For this review, take the finished solid that the model builds, in its own axes (mm). A direction names the side the tool comes from. Coordinates: 2 decimals unless noted, no trailing zeros. Loops run counter-clockwise (first coordinate to the right, second up) from the corner with the lowest first, then second, coordinate; pieces in that order, holes last. Notation, with made-up numbers: (9, 75.25) - (42, 75.25) arc R5 ccw to (42, 81.25) - close; hole circle Ø1 at (59.5, 36.25). An arc over 180 degrees is marked (long way). Use one line per item in the form item = value. Start each with the question number.
1. For pin 1 Ø8 at (x, z) = (80, 2) entering from +Y; pin 2 Ø6 at (x, y) = (89, -21) entering from +Z; pin 3 Ø3 at (y, z) = (-10.5, 16) entering from +X; pin 4 Ø8 at (x, z) = (128.5, -6) entering from +Y, all flat-tipped, find the tip position at first contact; note any pin that passes through.
2. Add section D-D on z = 19. Give the boundary of the cut face in (x, y).
3. To check wall thickness, follow probe 1 along X at (y, z) = (-9.5, 2); probe 2 along X at (y, z) = (31.5, 10.5); probe 3 along Z at (x, y) = (44, -8.5). State the ranges of each line that lie inside material, in increasing order.
4. Add section A-A on z = 0. Give the boundary of the cut face in (x, y).
5. Add section C-C on x = 13. Give the boundary of the cut face in (y, z), and give its area (3 significant figures).
6. Machinability: for faces 1 (the face through (137.1, -1.73, -7.81)), 2 (the face through (160.22, -2.17, -9.76)), 3 (the face through (60, 15, 0)), which of the approach directions +Z, -Z, +X, -X, +Y, -Y give a long, thin tool a straight path to every point of the face, cutting with its end or side? Answer none if there is none.
Autodesk Inventor part; units mm, degrees
ref_plane "YZ Plane" through (0, 0, 0) normal (1, 0, 0) x (0, 1, 0)
ref_plane "XZ Plane" through (0, 0, 0) normal (0, 1, 0) x (-1, 0, 0)
ref_plane "XY Plane" through (0, 0, 0) normal (0, 0, 1) x (1, 0, 0)
sketch "Sketch1" plane through (0, 0, 0) normal (0, 0, 1) x (1, 0, 0)
  line L0 (0, 0) -> (0, 13.5)
  line L1 (0, 13.5) -> (60, 13.5)
  line L2 (60, 13.5) -> (60, 0) construction
  line L3 (60, 0) -> (60, 34)
  line L4 (60, 34) -> (78, 34)
  line L5 (78, 34) -> (78, 0)
  line L6 (78, 0) -> (78, 21)
  line L7 (78, 21) -> (99, 21)
  line L8 (99, 21) -> (99, 0)
  line L9 (99, 0) -> (99, 15)
  line L10 (99, 15) -> (110, 15)
  line L11 (110, 15) -> (110, 0)
  line L12 (110, 0) -> (110, 10)
  line L13 (110, 10) -> (130, 10)
  line L14 (130, 10) -> (130, 0)
  line L15 (130, 0) -> (130, 8)
  line L16 (130, 8) -> (144, 8)
  line L17 (144, 8) -> (144, 0)
  line L18 (144, 0) -> (144, 10)
  line L19 (144, 10) -> (176, 10)
  line L20 (176, 10) -> (176, 0)
  line L21 (0, 0) -> (291.3618, 0) construction
  line L22 (0, 0) -> (176, 0)
  line L23 (47.9027, 0) -> (47.9027, 4) construction
  line L24 (60, 4) -> (56.5, 4) construction
  line L25 (52.5, 4) -> (40.5, 4)
  line L26 (36.5, 4) -> (33, 4) construction
  line L27 (33, 4) -> (0, 4) construction
  line L28 (46.5, 4) -> (46.5, 2) construction
  line L29 (46.5, 2) -> (40.5, 2) construction
  arc A0 (40.5, 4) -> (40.5, -4) centre (40.5, 0) ccw
  line L30 (46.5, 2) -> (52.5, 2) construction
  arc A1 (52.5, -4) -> (52.5, 4) centre (52.5, 0) ccw
  line L31 (40.5, -4) -> (52.5, -4)
  dimension "d4" = 13.5
  dimension "d5" = 60
  dimension "d9" = 18
  dimension "d10" = 21
  dimension "d11" = 21
  dimension "d12" = 15
  dimension "d13" = 11
  dimension "d14" = 10
  dimension "d15" = 20
  dimension "d16" = 8
  dimension "d17" = 14
  dimension "d18" = 10
  dimension "d19" = 32
  dimension "d28" = 3.5
  dimension "d29" = 20
  dimension "d30" = 3.5
  dimension "d31" = 6
  dimension "d32" = 8
  dimension "d33" = 6
  dimension "d34" = 8
revolve "Revolution1" add sketch "Sketch1" angle 360 about axis through (0, 0, 0) along (1, 0, 0) contours L0 L1 L3 L22 A1 L25 A0 | A0 L25 A1 L22 | L3 L4 L5 L22 | L5 L7 L8 L22 | L8 L10 L11 L22 | L11 L13 L14 L22 | L14 L16 L17 L22 | L17 L18 L19 L20 L22
sketch "Sketch2" plane through (0, 0, 0) normal (-1, 0, 0) x (0, 0, 1)
  circle A0 centre (0, 0) radius 13.5
  line L0 (-13.5, 0) -> (9.5, 0) construction
  line L1 (9.5, 0) -> (9.5, 4) construction
  line L2 (9.5, 0) -> (9.5, -4) construction
  dimension "d21" = 23
  dimension "d22" = 4
  dimension "d23" = 4
Conclusion:
q1.pin_1 = 34
q1.pin_2 = 10.82
q1.pin_3 = 99
q1.pin_4 = 9.8
q2.outline = (60, -28.2) - (78, -28.2) - (78, -8.94) - (99, -8.94) - (99, 8.94) - (78, 8.94) - (78, 28.2) - (60, 28.2) - close
q3.probe_1 = 0 to 130, 144 to 176
q3.probe_2 = 60 to 78
q3.probe_3 = -10.49 to 10.49
q4.outline = (0, -13.5) - (60, -13.5) - (60, -34) - (78, -34) - (78, -21) - (99, -21) - (99, -15) - (110, -15) - (110, -10) - (130, -10) - (130, -8) - (144, -8) - (144, -10) - (176, -10) - (176, 10) - (144, 10) - (144, 8) - (130, 8) - (130, 10) - (110, 10) - (110, 15) - (99, 15) - (99, 21) - (78, 21) - (78, 34) - (60, 34) - (60, 13.5) - (0, 13.5) - close
q5.outline = circle Ø27 at (0, 0)
q5.area = 573 mm^2
q6.face_1 = none
q6.face_2 = +X
q6.face_3 = -X
